from build123d import *

# Parameters (mm, degrees)
F0_R     = 12.5
F0_R_2   = 2.15
F0_W     = 3
F0_H     = 6
F0_R_3   = 2.585
F1_DEPTH = 6
F0_R_4   = 1.65
F2_DEPTH = 1
F3_R     = 1.75
F4_DEPTH = 12.5
F5_START = -10
F3_R_2   = 3.2
F5_DEPTH = 15
F6_START = 10
F6_DEPTH = 15


with BuildPart() as f1:
    # F0 (on Top) → F1 (new body)
    with BuildSketch(Plane.XY):
        Circle(F0_R)
        with Locations((0, -9)):
            Circle(F0_R_2, mode=Mode.SUBTRACT)
        with Locations((-6, 0)):
            Rectangle(F0_W, F0_H, mode=Mode.SUBTRACT)
        Circle(F0_R_3, mode=Mode.SUBTRACT)
        with Locations((6, 0)):
            Rectangle(F0_W, F0_H, mode=Mode.SUBTRACT)
        with Locations((0, 9)):
            Circle(F0_R_2, mode=Mode.SUBTRACT)
        Circle(F0_R)
        with Locations((0, -9)):
            Circle(F0_R_2, mode=Mode.SUBTRACT)
        with Locations((-6, 0)):
            Rectangle(F0_W, F0_H, mode=Mode.SUBTRACT)
        Circle(F0_R_3, mode=Mode.SUBTRACT)
        with Locations((6, 0)):
            Rectangle(F0_W, F0_H, mode=Mode.SUBTRACT)
        with Locations((0, 9)):
            Circle(F0_R_2, mode=Mode.SUBTRACT)
    extrude(amount=F1_DEPTH)

    # F0 (on Top) → F2 (join)
    with BuildSketch(Plane.XY):
        with Locations((0, 9)):
            Circle(F0_R_2)
        with Locations((0, 9)):
            Circle(F0_R_4, mode=Mode.SUBTRACT)
        with Locations((0, -9)):
            Circle(F0_R_2)
        with Locations((0, -9)):
            Circle(F0_R_4, mode=Mode.SUBTRACT)
    extrude(amount=F2_DEPTH)

    # F3 (on Right) → F4 (cut, symmetric)
    with BuildSketch(Plane.YZ):
        with Locations((0, 3)):
            Circle(F3_R)
    extrude(amount=F4_DEPTH, both=True, mode=Mode.SUBTRACT)

    # F3 (on Right) → F5 (cut)
    with BuildSketch(Plane.YZ.offset(F5_START)):
        with Locations((0, 3)):
            Circle(F3_R_2)
        with Locations((0, 3)):
            Circle(F3_R, mode=Mode.SUBTRACT)
    extrude(amount=-F5_DEPTH, mode=Mode.SUBTRACT)

    # F3 (on Right) → F6 (cut)
    with BuildSketch(Plane.YZ.offset(F6_START)):
        with Locations((0, 3)):
            Circle(F3_R_2)
        with Locations((0, 3)):
            Circle(F3_R, mode=Mode.SUBTRACT)
    extrude(amount=F6_DEPTH, mode=Mode.SUBTRACT)


solid = f1.part
Build history of the part. All positions in model axes, mm. A direction names the side the tool comes from. Round coordinates to 2 decimals unless told otherwise and drop trailing zeros. Write each loop counter-clockwise with the first axis right and the second up, starting at its lowest first coordinate (ties: lowest second). Pieces come first, ordered by that corner, then holes. Notation, with made-up numbers: M 42.5,79.25 L 52.5,79.25 A6 cw 52.5,89.25 Z; hole C 60.25,10.25 d7. An arc over 180 degrees is marked long. Answer in a Markdown table with one row per item.
1. Saw through at A-A (x = 0). List the corners of the cut face in (y, z) (3 decimals), and give its area (3 significant figures).
Geometry check:
| item | result |
|---|---|
| outline | M -12.5,0 L -10.65,0 L -10.65,1 L -11.15,1 L -11.15,6 L -12.5,6 Z; M -7.35,0 L -2.585,0 L -2.585,6 L -6.85,6 L -6.85,1 L -7.35,1 Z; M 2.585,0 L 7.35,0 L 7.35,1 L 6.85,1 L 6.85,6 L 2.585,6 Z; M 10.65,0 L 12.5,0 L 12.5,6 L 11.15,6 L 11.15,1 L 10.65,1 Z |
| area | 69.4 mm2 |
2. Flat gauge pins, fed straight in: P1, Ø2, axis at y = 8.5, z = 2, coming from the +X side; P2, Ø2.5, axis at x = -6.5, z = 2, coming from the +Y side; P3, Ø1.8, axis at y = 1.5, z = 2.5, coming from the -X side. Where does each tip first touch, or does it go through?
Geometry check:
| item | result |
|---|---|
| P1 | x = 10 |
| P2 | y = 11.34 |
| P3 | x = -10 |
3. Saw through at D-D (x = 5.75). List the corners of the cut face in (y, z).
Geometry check:
| item | result |
|---|---|
| outline | M -11.1,0 L -3,0 L -3,6 L -11.1,6 Z; M 3,0 L 11.1,0 L 11.1,6 L 3,6 Z |
4. Which spindle directions (+Z, -Z, +X, -X, +Y, -Y) get a long thin tool onto all of the face, cutting with end or side? Do faces 1 (the face through (-11.2, 3.2, 2.9)), 2 (the face through (-0.28, -6.87, 3.46)), 3 (the face through (10, 1.4, 4.4)), 4 (the face through (-6, -3, 3)). Say none if no direction does.
Geometry check:
| item | result |
|---|---|
| face 1 | -X |
| face 2 | +Z |
| face 3 | +X |
| face 4 | +Z, -Z |
5. Probe L1, parallel to Y at x = 0, z = 2.5 (3 decimals); L2, parallel to Y at x = 0.5, z = 2.25; L3, parallel to Y at x = -3.25, z = 2.75. List the from-to ranges inside material, lowest first. Write a range as [from, to].
Geometry check:
| item | result |
|---|---|
| L1 | [-12.5, -11.15], [-6.85, -2.585], [2.585, 6.85], [11.15, 12.5] |
| L2 | [-12.49, -11.09], [-6.91, -2.54], [2.54, 6.91], [11.09, 12.49] |
| L3 | [-12.07, -1.73], [1.73, 12.07] |
6. Mould opens along Z. For faces 5 (the face through (3.508, 1.617, 2.33)), 6 (the face through (0, -11, 1)), 7 (the face through (6, 3, 3)) say: +Z half, -Z half, draft (parallel to the pull), parting line (faces both ways), or undercut.
Geometry check:
| item | result |
|---|---|
| face 5 | undercut |
| face 6 | +Z half |
| face 7 | draft |
7. Saw through at B-B (z = 4.25). State how many separate pieces and enclosed holes the cut face has, and give its area (3 significant figures).
Geometry check:
| item | result |
|---|---|
| separate pieces | 2 |
| enclosed holes | 2 |
| area | 355 mm2 |
